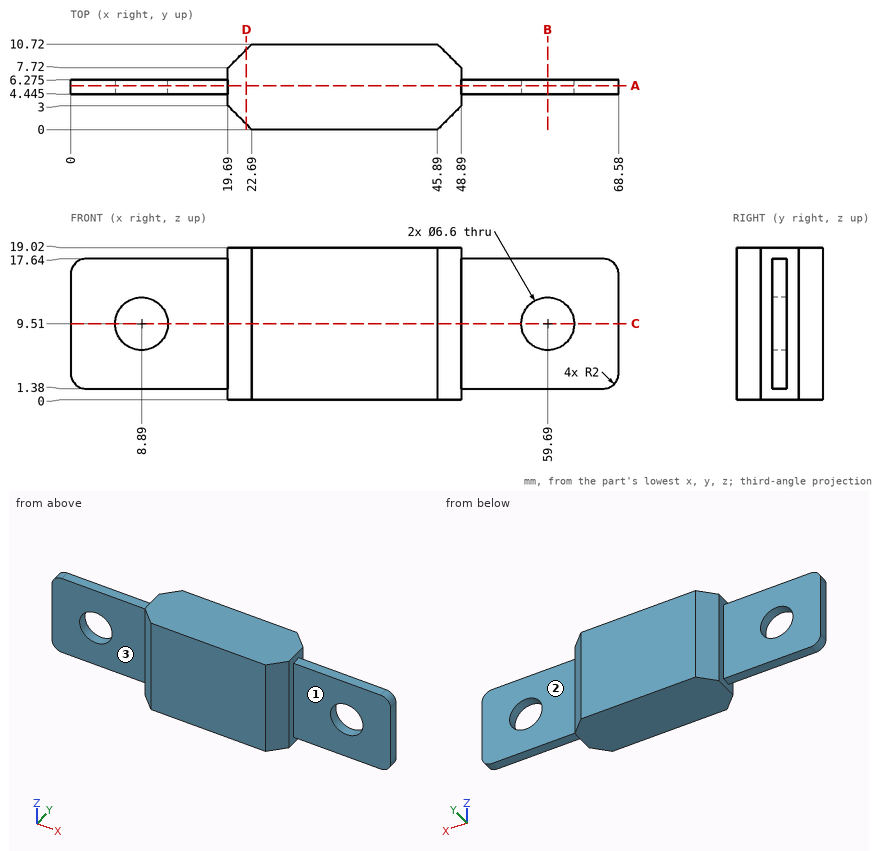
Design review of the part shown in the three views and the two pictorial views. Dimensions are in mm from the part's minimum x, y and z. A direction names the side the tool comes from. Give positions to 0.01 mm unless a question says otherwise; leave off trailing zeros. Loops run counter-clockwise (first coordinate to the right, second up) from the corner with the lowest first, then second, coordinate; pieces in that order, holes last. Notation, with made-up numbers: (-1, -5.5) -> (43, -5.5) arc R5 cw to (43, 0.5) -> close; hole circle Ø5 at (-15.75, 32). An arc over 180 degrees is marked (long way). Answer as a JSON object with one key per item and string values. Group by question number.
Q1. Take a section at D-D (x = 22). Write out the cut boundary in (y, z), plus the area to 3 significant figures.
Q2. Tool access review of the marked faces 1, 2 and 3: name each direction out of +Z, -Z, +X, -X, +Y, -Y from which nothing blocks a thin tool from reaching the whole face with its end or side.
Q3. Insertion check: pin 1 (3 mm diameter, centred on x = 58, y = 7.5, fed in from -Z); pin 2 (8 mm diameter, centred on x = 61.5, z = 5.5, fed in from -Y) (3 decimals); pin 3 (1.5 mm diameter, centred on x = 60.5, y = 5.5, fed in from +Z). Each pin has a flat end and moves straight along its axis. Give the tip position at first contact, or say it passes through.
Q4. Take a section at C-C (z = 9.51). Write out the cut boundary in (x, y) (3 decimals).
Q5. Wall thickness on line 1 along X through (y, z) = (5.6, 9.51); line 2 along Z through (x, y) = (59.69, 5.15); line 3 along X through (y, z) = (4.5, 7.5): over which ranges is each line inside the solid? List them lowest first.
Q6. Take a section at B-B (x = 59.69). Write out the cut boundary in (y, z) (3 decimals).
Q7. Take a section at A-A (y = 5.5). Write out the cut boundary in (x, z), plus the area to 3 significant figures.
Answer below:
{
 "1": {"outline": "(0.69, 0) -> (10.03, 0) -> (10.03, 19.02) -> (0.69, 19.02) -> close", "area": "178 mm2"},
 "2": {"face 1": "+Z, -Z, +X, -Y", "face 2": "+Z, -Z, +X, +Y", "face 3": "+Z, -Z, -X, -Y"},
 "3": {"pin 1": "stops at z = 1.38", "pin 2": "stops at y = 4.445", "pin 3": "stops at z = 17.64"},
 "4": {"outline": "(0, 4.445) -> (5.59, 4.445) -> (5.59, 6.275) -> (0, 6.275) -> close; (12.19, 4.445) -> (19.69, 4.445) -> (19.69, 3) -> (22.69, 0) -> (45.89, 0) -> (48.89, 3) -> (48.89, 4.445) -> (56.39, 4.445) -> (56.39, 6.275) -> (48.89, 6.275) -> (48.89, 7.72) -> (45.89, 10.72) -> (22.69, 10.72) -> (19.69, 7.72) -> (19.69, 6.275) -> (12.19, 6.275) -> close; (62.99, 4.445) -> (68.58, 4.445) -> (68.58, 6.275) -> (62.99, 6.275) -> close"},
 "5": {"line 1": "x = 0 to 5.59, 12.19 to 56.39, 62.99 to 68.58", "line 2": "z = 1.38 to 6.21, 12.81 to 17.64", "line 3": "x = 0 to 6.27, 11.51 to 57.07, 62.31 to 68.58"},
 "6": {"outline": "(4.445, 1.38) -> (6.275, 1.38) -> (6.275, 6.21) -> (4.445, 6.21) -> close; (4.445, 12.81) -> (6.275, 12.81) -> (6.275, 17.64) -> (4.445, 17.64) -> close"},
 "7": {"outline": "(0, 3.38) arc R2 ccw to (2, 1.38) -> (19.69, 1.38) -> (19.69, 0) -> (48.89, 0) -> (48.89, 1.38) -> (66.58, 1.38) arc R2 ccw to (68.58, 3.38) -> (68.58, 15.64) arc R2 ccw to (66.58, 17.64) -> (48.89, 17.64) -> (48.89, 19.02) -> (19.69, 19.02) -> (19.69, 17.64) -> (2, 17.64) arc R2 ccw to (0, 15.64) -> close; hole circle Ø6.6 at (8.89, 9.51); hole circle Ø6.6 at (59.69, 9.51)", "area": "1,120 mm2"}
}
